The listing builds one solid part. Answer for the finished solid, in the listing's coordinates (mm). A direction names the side the tool comes from. Give positions to 0.01 mm unless a question says otherwise; leave off trailing zeros. Order: outer loops, then holes, each group sorted by start corner. A loop starts at its lowest first (then second) coordinate and runs counter-clockwise, first axis right, second up. Notation, with made-up numbers: (70.25, 79) - (108.25, 79) arc R14 cw to (108.25, 89) - close; hole circle Ø9 at (-17, 84). An arc over 180 degrees is marked (long way). Use a Markdown table: item, result. Add a question column.
1) Find section B-B, the plane z = -14. State how many separate pieces and enclosed holes the cut face has, plus the area to 3 significant figures.
2) Find section A-A, the plane y = 96. Determine the outline of the cut face in (x, z).
3) For faces 1 (the face through (117.177, 149, -14)), 2 (the face through (275, 88, -18)), 3 (the face through (237, 26.2, -18)), determine the directions among +Z, -Z, +X, -X, +Y, -Y from which every point of the face is accessible in a straight line to the end or side of a thin tool.
4) The mould has two halves that part along X. Classify faces 4 (the face through (-69.466, -42.916, -14.423)), 5 (the face through (237, -68.8, -18)), 6 (the face through (-165.823, 116, -14)), 7 (the face through (200, 136, -18)): released by +X, released by -X, zero draft, split by the parting line, or undercut.
5) Flat-ended cylindrical pins translate along their axes: pin 1 (4 mm diameter, centred on x = 225, y = 0, fed in from +Z); pin 2 (8 mm diameter, centred on y = -44, z = -17.5, fed in from +X). Find the tip coordinate at first contact, or state that the pin passes through.
6) Straight lines are drawn through the part: line 1 (Y direction, x = -255, z = -17); line 2 (Y direction, x = 215, z = -15.75); line 3 (Y direction, x = 236.5, z = -23.25). For each, find the intervals that lie inside material, in ascending order.
from build123d import *

# Parameters (mm, degrees)
SKETCH011_W     = 550
SKETCH011_H     = 350
PAD012_DEPTH    = 19
SKETCH012_R     = 4
POCKET007_DEPTH = 11
FILLET_R        = 20
SKETCH013_R     = 2
POCKET008_DEPTH = 19.001
SKETCH014_W     = 75
SKETCH014_H     = 30
POCKET009_DEPTH = 19.001
FILLET004_R     = 6
SKETCH028_R     = 2
POCKET018_DEPTH = 19.001
CHAMFER008_SIZE = 6


with BuildPart() as part:
    # Sketch011 → Pad012 (new body)
    with BuildSketch(Plane.XY):
        with Locations((0, 41.2)):
            Rectangle(SKETCH011_W, SKETCH011_H)
    extrude(amount=-PAD012_DEPTH)

    # Sketch012 (on Face5 of Pad012) → Pocket007 (cut)
    with BuildSketch(Plane.XY):
        with Locations((-238, 0)):
            Circle(SKETCH012_R)
        with Locations((225, 0)):
            Circle(SKETCH012_R)
        with BuildLine():
            ThreePointArc((-165.823184, 24.404903), (-159.323184, 17.904903), (-152.823184, 24.404903))
            Line((-152.823184, 24.404903), (-152.823184, 216.2))
            ThreePointArc((-152.823184, 216.2), (-159.323184, 222.7), (-165.823184, 216.2))
            Line((-165.823184, 24.404903), (-165.823184, 216.2))
        make_face()
        with BuildLine():
            ThreePointArc((-75.823184, -36.417713), (-69.323184, -42.917713), (-62.823184, -36.417713))
            Line((-62.823184, -36.417713), (-62.823184, 216.2))
            ThreePointArc((-62.823184, 216.2), (-69.323184, 222.7), (-75.823184, 216.2))
            Line((-75.823184, -36.417713), (-75.823184, 216.2))
        make_face()
        with BuildLine():
            ThreePointArc((14.176816, 28.977719), (20.676816, 22.477719), (27.176816, 28.977719))
            Line((27.176816, 28.977719), (27.176816, 216.2))
            ThreePointArc((27.176816, 216.2), (20.676816, 222.7), (14.176816, 216.2))
            Line((14.176816, 28.977719), (14.176816, 216.2))
        make_face()
        with BuildLine():
            ThreePointArc((104.176816, 89.800335), (110.676816, 83.300335), (117.176816, 89.800335))
            Line((117.176816, 89.800335), (117.176816, 216.2))
            ThreePointArc((117.176816, 216.2), (110.676816, 222.7), (104.176816, 216.2))
            Line((104.176816, 89.800335), (104.176816, 216.2))
        make_face()
    extrude(amount=-POCKET007_DEPTH, mode=Mode.SUBTRACT)

    # Fillet
    fillet_edges = [part.edges().sort_by_distance(p)[0] for p in [
        (-275, -133.8, -9.5),
        (-275, 216.2, -9.5),
    ]]
    fillet(fillet_edges, radius=FILLET_R)

    # Sketch013 (on Face2 of Fillet) → Pocket008 (cut, through all)
    with BuildSketch(Plane.XY):
        with Locations((-255, 196.2)):
            Circle(SKETCH013_R)
        with Locations((-255, -113.8)):
            Circle(SKETCH013_R)
        with Locations((215, -113.8)):
            Circle(SKETCH013_R)
        with Locations((215, 196.2)):
            Circle(SKETCH013_R)
    extrude(amount=-POCKET008_DEPTH, mode=Mode.SUBTRACT)

    # Sketch014 (on Face2 of Pocket008) → Pocket009 (cut, through all)
    with BuildSketch(Plane.XY):
        with Locations((237.5, 136.2)):
            Rectangle(SKETCH014_W, SKETCH014_H)
        with Locations((237.5, -53.8)):
            Rectangle(SKETCH014_W, SKETCH014_H)
        with Locations((237.5, 41.2)):
            Rectangle(SKETCH014_W, SKETCH014_H)
    extrude(amount=-POCKET009_DEPTH, mode=Mode.SUBTRACT)

    # Fillet004
    fillet004_edges = [part.edges().sort_by_distance(p)[0] for p in [
        (275, 151.2, -9.5),
        (200, 151.2, -9.5),
        (275, 121.2, -9.5),
        (275, 56.2, -9.5),
        (200, 56.2, -9.5),
        (275, 26.2, -9.5),
        (200, -38.8, -9.5),
        (275, -38.8, -9.5),
        (275, -68.8, -9.5),
        (200, -68.8, -9.5),
        (200, 26.2, -9.5),
        (200, 121.2, -9.5),
    ]]
    fillet(fillet004_edges, radius=FILLET004_R)

    # Sketch028 (on Face50 of Fillet004) → Pocket018 (cut, through all)
    with BuildSketch(Plane(origin=(0, 0, -19), x_dir=(1, 0, 0), z_dir=(0, 0, -1))):
        with Locations((255, -196.2)):
            Circle(SKETCH028_R)
        with Locations((255, 113.8)):
            Circle(SKETCH028_R)
    extrude(amount=-POCKET018_DEPTH, mode=Mode.SUBTRACT)

    # Chamfer008
    chamfer008_edges = [part.edges().sort_by_distance(p)[0] for p in [
        (-165.823184, 216.2, -5.5),
        (-152.823184, 216.2, -5.5),
        (-75.823184, 216.2, -5.5),
        (-62.823184, 216.2, -5.5),
        (14.176816, 216.2, -5.5),
        (27.176816, 216.2, -5.5),
        (104.176816, 216.2, -5.5),
        (117.176816, 216.2, -5.5),
    ]]
    chamfer(chamfer008_edges, length=CHAMFER008_SIZE)


with BuildPart() as part_1:
    # Body008 placement: moved
    add(part.part.moved(Location((0, 0, -9))))


solid = part_1.part
The answers:
| question | item | result |
|---|---|---|
| 1 | separate pieces | 1 |
| 1 | enclosed holes | 8 |
| 1 | area | 175,000 mm2 |
| 2 | outline | (-275, -28) - (275, -28) - (275, -9) - (117.18, -9) - (117.18, -20) - (104.18, -20) - (104.18, -9) - (27.18, -9) - (27.18, -20) - (14.18, -20) - (14.18, -9) - (-62.82, -9) - (-62.82, -20) - (-75.82, -20) - (-75.82, -9) - (-152.82, -9) - (-152.82, -20) - (-165.82, -20) - (-165.82, -9) - (-275, -9) - close |
| 3 | face 1 | +Z, +Y |
| 3 | face 2 | +Z, -Z, +X, +Y, -Y |
| 3 | face 3 | +Z, -Z, +X |
| 4 | face 4 | undercut |
| 4 | face 5 | zero draft |
| 4 | face 6 | undercut |
| 4 | face 7 | released by +X |
| 5 | pin 1 | z = -20 |
| 5 | pin 2 | x = 202.4 |
| 6 | line 1 | -133.8 to -115.8, -111.8 to 194.2, 198.2 to 216.2 |
| 6 | line 2 | -133.8 to -115.8, -111.8 to -68.8, -38.8 to 26.2, 56.2 to 121.2, 151.2 to 194.2, 198.2 to 216.2 |
| 6 | line 3 | -133.8 to -68.8, -38.8 to 26.2, 56.2 to 121.2, 151.2 to 216.2 |
